```python
from build123d import *

# Parameters (mm, degrees)
SKETCH1_R           = 74
SKETCH1_R_2         = 2.55
BOSS_EXTRUDE1_DEPTH = 3.5
SKETCH2_R           = 32.5
SKETCH2_R_2         = 16
CUT_EXTRUDE4_DEPTH  = 1
FILLET1_R           = 1.5
FILLET2_R           = 1.5
SKETCH3_R           = 74
SKETCH3_R_2         = 72
BOSS_EXTRUDE2_DEPTH = 25.4
CUT_EXTRUDE5_START  = -15
CUT_EXTRUDE5_DEPTH  = 15
CIRPATTERN2_COUNT   = 4
FILLET4_R           = 1.5
SKETCH6_R           = 0.75
BOSS_EXTRUDE3_DEPTH = 17


with BuildPart() as part:
    # Sketch1 → Boss-Extrude1 (new body)
    with BuildSketch(Plane.XY):
        Circle(SKETCH1_R)
        Circle(SKETCH1_R_2, mode=Mode.SUBTRACT)
    extrude(amount=BOSS_EXTRUDE1_DEPTH)

    # Sketch2 → Cut-Extrude4 (cut)
    with BuildSketch(Plane.XY):
        Circle(SKETCH2_R)
        Circle(SKETCH2_R_2, mode=Mode.SUBTRACT)
    extrude(amount=CUT_EXTRUDE4_DEPTH, mode=Mode.SUBTRACT)

    # Fillet1
    # the kernel refuses this fillet: 1.5 mm, written as the material it takes off along each edge
    with BuildSketch(Plane(origin=(0, 0, 0), x_dir=(1, 0, 0), z_dir=(0, -1, 0))) as fillet1_piece_1:
        with BuildLine():
            CenterArc((33.914213562, 1.5), FILLET1_R, 199.471220634, 70.528779366)
            Line((32.5, 1), (32.471715729, 0.99))
            ThreePointArc((32.471715729, 0.99), (32.47, 0.5), (32.47, 0))
            Line((32.47, 0), (32.5, -0.03))
            Line((32.5, -0.03), (33.914213562, -0.03))
            Line((33.914213562, -0.03), (33.914213562, 0))
        make_face()
    revolve(axis=Axis((0, 0, 0), (0, 0, 1)), mode=Mode.SUBTRACT)

    # Fillet2
    # the kernel refuses this fillet: 1.5 mm, written as the material it takes off along each edge
    with BuildSketch(Plane(origin=(0, 0, 0), x_dir=(1, 0, 0), z_dir=(0, -1, 0))) as fillet2_piece_1:
        with BuildLine():
            CenterArc((14.585786438, 1.5), FILLET2_R, 270, 70.528779366)
            Line((16, 1), (16.028284271, 0.99))
            ThreePointArc((16.028284271, 0.99), (16.03, 0.5), (16.03, 0))
            Line((16.03, 0), (16, -0.03))
            Line((16, -0.03), (14.585786438, -0.03))
            Line((14.585786438, -0.03), (14.585786438, 0))
        make_face()
    revolve(axis=Axis((0, 0, 0), (0, 0, 1)), mode=Mode.SUBTRACT)

    # Sketch3 → Boss-Extrude2 (add)
    with BuildSketch(Plane.XY):
        Circle(SKETCH3_R)
        Circle(SKETCH3_R_2, mode=Mode.SUBTRACT)
    extrude(amount=BOSS_EXTRUDE2_DEPTH)

    # Sketch5 → Cut-Extrude5 (cut)
    with BuildSketch(Plane.XY.offset(25.4).offset(CUT_EXTRUDE5_START)):
        with BuildLine():
            Line((-12.354120349, 70.932190932), (-12.697290359, 72.902529569))
            ThreePointArc((-12.697290359, 72.902529569), (0.361150189, 73.999118715), (13.408265197, 72.775122291))
            Line((13.408265197, 72.775122291), (13.045879651, 70.808227094))
            ThreePointArc((13.045879651, 70.808227094), (0.351389373, 71.999142533), (-12.354120349, 70.932190932))
        make_face()
    cut_extrude5 = extrude(amount=CUT_EXTRUDE5_DEPTH, mode=Mode.SUBTRACT)

    # CirPattern2: Cut-Extrude5 ×4 about axis
    cirpattern2_axis = Axis((0, 0, 0), (0, 0, -1))
    for i in range(1, CIRPATTERN2_COUNT):
        add(cut_extrude5.rotate(cirpattern2_axis, i * 360 / CIRPATTERN2_COUNT), mode=Mode.SUBTRACT)

    # Fillet4
    fillet4_edges = [part.edges().sort_by_distance(p)[0] for p in [
        (13.227072424, 71.791674692, 10.4),
        (-12.525705354, 71.91736025, 10.4),
        (-71.791674692, 13.227072424, 10.4),
        (-71.91736025, -12.525705354, 10.4),
        (-13.227072424, -71.791674692, 10.4),
        (12.525705354, -71.91736025, 10.4),
        (71.791674692, -13.227072424, 10.4),
        (71.91736025, 12.525705354, 10.4),
    ]]
    fillet(fillet4_edges, radius=FILLET4_R)

    # Sketch6 → Boss-Extrude3 (add)
    with BuildSketch(Plane.XY.offset(3.5)):
        with Locations((18, 28)):
            Circle(SKETCH6_R)
        with Locations((-18, 28)):
            Circle(SKETCH6_R)
        with Locations((-18, -28)):
            Circle(SKETCH6_R)
        with Locations((18, -28)):
            Circle(SKETCH6_R)
    extrude(amount=BOSS_EXTRUDE3_DEPTH)


solid = part.part
```
Build history of the part. All positions in model axes, mm. A direction names the side the tool comes from. Round coordinates to 2 decimals unless told otherwise and drop trailing zeros. Write each loop counter-clockwise with the first axis right and the second up, starting at its lowest first coordinate (ties: lowest second). Pieces come first, ordered by that corner, then holes. Notation, with made-up numbers: (27.5, -12.5) - (50.5, -12.5) arc R15 cw to (50.5, 0.5) - close; hole circle Ø7 at (-11, -16.5). An arc over 180 degrees is marked (long way). Write each question's results on one line, items separated by ' | '. Start each with the question number.
Item 1: Drop flat-ended pins along their axis: P1, Ø3, axis at x = -4.5, y = -72.5, coming from the +Z side; P2, Ø1.2, axis at x = -18, y = 27.5, coming from the +Z side; P3, Ø5, axis at x = 35.5, y = -45, coming from the +Z side. Give the stop position or say it passes through.
Item 2: Saw through at B-B (y = 0). Write the cut outline in (x, z), and give its area (3 significant figures).
Item 3: Saw through at D-D (x = -42.5). Write the cut outline in (y, z), and give its area (3 significant figures).
Item 4: Mould opens along X. For faces 1 (the face through (32, -15, 0)), 2 (the face through (68.36, -28.34, 12.52)), 3 (the face through (1.18, -2.26, 1.73)) say: pulls with the +X half, pulls with the -X half, needs draft (parallel to the pull), parting line crosses it, or undercut.
Item 5: Wall check: L1, parallel to Y at x = 0, z = 2.05; L2, parallel to Z at x = -17, y = -26; L3, parallel to Z at x = -25.5, y = 64. Give the ranges that are in metal, low to high. Write a range as [from, to].
Item 6: Saw through at A-A (z = 6.25). Write the cut outline in (x, y).
Item 7: Saw through at C-C (z = 14). Write the cut outline in (x, y).
Item 8: Which spindle directions (+Z, -Z, +X, -X, +Y, -Y) get a long thin tool onto all of the face, cutting with end or side? Do faces 4 (the face through (-52, 52, 25.4)), 5 (the face through (66.5, -27.6, 14.3)), 6 (the face through (7, 15, 1)). Say none if no direction does.
Results are:
1) P1: stops at z = 10.4 | P2: stops at z = 20.5 | P3: stops at z = 3.5
2) outline: (-74, 0) - (-33.91, 0) arc R1.5 ccw to (-32.5, 1) - (-16, 1) arc R1.5 ccw to (-14.59, 0) - (-2.55, 0) - (-2.55, 3.5) - (-72, 3.5) - (-72, 10.4) - (-74, 10.4) - close; (2.55, 0) - (14.59, 0) arc R1.5 ccw to (16, 1) - (32.5, 1) arc R1.5 ccw to (33.91, 0) - (74, 0) - (74, 10.4) - (72, 10.4) - (72, 3.5) - (2.55, 3.5) - close | area: 493 mm²
3) outline: (-60.58, 0) - (60.58, 0) - (60.58, 25.4) - (58.12, 25.4) - (58.12, 3.5) - (-58.12, 3.5) - (-58.12, 25.4) - (-60.58, 25.4) - close | area: 532 mm²
4) face 1: needs draft | face 2: parting line crosses it | face 3: undercut
5) L1: y = [-74, -2.55], [2.55, 74] | L2: z = [1, 3.5] | L3: z = [0, 3.5]
6) outline: circle Ø148 at (0, 0); circle Ø1.5 at (-18, -28); circle Ø1.5 at (-18, 28); circle Ø1.5 at (18, -28); circle Ø1.5 at (18, 28); hole circle Ø144 at (0, 0)
7) outline: (-72.9, -12.7) arc R74 ccw to (-13.41, -72.78) - (-13.05, -70.81) arc R72 cw to (-70.93, -12.35) - close; (-72.78, 13.41) - (-70.81, 13.05) arc R72 cw to (-12.35, 70.93) - (-12.7, 72.9) arc R74 ccw to start; circle Ø1.5 at (-18, -28); circle Ø1.5 at (-18, 28); (12.35, -70.93) - (12.7, -72.9) arc R74 ccw to (72.78, -13.41) - (70.81, -13.05) arc R72 cw to start; (13.05, 70.81) arc R72 cw to (70.93, 12.35) - (72.9, 12.7) arc R74 ccw to (13.41, 72.78) - close; circle Ø1.5 at (18, -28); circle Ø1.5 at (18, 28)
8) face 4: +Z, +X, -X, +Y, -Y | face 5: +Z | face 6: -Z
